from build123d import *

# Parameters (mm, degrees)
SKETCH1_W           = 92.252714028
SKETCH1_H           = 52.835645306
SKETCH1_R           = 8.1
BOSS_EXTRUDE1_DEPTH = 3
SKETCH2_R           = 11.1
SKETCH2_R_2         = 8.1
BOSS_EXTRUDE2_DEPTH = 2


with BuildPart() as part:
    # Sketch1 → Boss-Extrude1 (new body)
    with BuildSketch(Plane(origin=(0, 0, 0), x_dir=(1, 0, 0), z_dir=(0, 1, 0))):
        Rectangle(SKETCH1_W, SKETCH1_H)
        with Locations(Location((-25.470998192, 0, 0), (0, 0, 270))):
            Circle(SKETCH1_R, mode=Mode.SUBTRACT)
    extrude(amount=BOSS_EXTRUDE1_DEPTH)

    # Sketch2 → Boss-Extrude2 (add)
    with BuildSketch(Plane(origin=(0, 3, 0), x_dir=(1, 0, 0), z_dir=(0, 1, 0))):
        with Locations(Location((-25.470998192, 0, 0), (0, 0, 90))):
            Circle(SKETCH2_R)
        with Locations(Location((-25.470998192, 0, 0), (0, 0, 270))):
            Circle(SKETCH2_R_2, mode=Mode.SUBTRACT)
    extrude(amount=BOSS_EXTRUDE2_DEPTH)


solid = part.part
Work out the finished part from the listing and answer in its coordinate system (mm). Round coordinates to 2 decimals unless told otherwise and drop trailing zeros. Write each loop counter-clockwise with the first axis right and the second up, starting at its lowest first coordinate (ties: lowest second). Pieces come first, ordered by that corner, then holes.
1) The mould has two halves that part along Z. Classify faces 1 (the flat face through (-1, 1, -26.418)), 2 (the cylindrical face through (-14.635, 3.986, 2.406)), 3 (the cylindrical face through (-32.657, 2.465, 3.738)), 4 (the flat face through (-46.126, 1, 0)): pulls with the +Z half, pulls with the -Z half, needs draft (parallel to the pull), parting line crosses it, or undercut.
2) A cutting plane is placed at C-C (y = 2). Give the vertices of the cut face in (x, z), plus the area to 3 significant figures.
3) Given pin 1 Ø1.5 at (x, z) = (4.5, -9.5) entering from +Y; pin 2 Ø13 at (x, z) = (-25.47, 0) entering from -Y, each flat-ended and moving along its own axis, determine where each tip first touches the part or whether it passes through.
4) A cutting plane is placed at A-A (z = 0). Give the vertices of the cut face in (x, y), plus the area to 3 significant figures.
5) A cutting plane is placed at B-B (x = -32). Give the vertices of the cut face in (y, z).
6) A cutting plane is placed at D-D (z = 22). Give the vertices of the cut face in (x, y), plus the area to 3 significant figures.
7) Straight lines are drawn through the part: line 1 (X direction, y = 2.2, z = 0); line 2 (X direction, y = 3.5, z = 0); line 3 (Y direction, x = -19, z = -24). For each, find the intervals that lie inside material, in ascending order.
Completed:
1. face 1: pulls with the -Z half
1. face 2: parting line crosses it
1. face 3: undercut
1. face 4: needs draft
2. outline: (-46.13, -26.42) - (46.13, -26.42) - (46.13, 26.42) - (-46.13, 26.42) - close; hole circle Ø16.2 at (-25.47, 0)
2. area: 4,670 mm2
3. pin 1: stops at y = 3
3. pin 2: passes through
4. outline: (-46.13, 0) - (-33.57, 0) - (-33.57, 5) - (-36.57, 5) - (-36.57, 3) - (-46.13, 3) - close; (-17.37, 0) - (46.13, 0) - (46.13, 3) - (-14.37, 3) - (-14.37, 5) - (-17.37, 5) - close
4. area: 240 mm2
5. outline: (0, -26.42) - (3, -26.42) - (3, -8.98) - (5, -8.98) - (5, -4.79) - (0, -4.79) - close; (0, 4.79) - (5, 4.79) - (5, 8.98) - (3, 8.98) - (3, 26.42) - (0, 26.42) - close
6. outline: (-46.13, 0) - (46.13, 0) - (46.13, 3) - (-46.13, 3) - close
6. area: 277 mm2
7. line 1: x = -46.13 to -33.57, -17.37 to 46.13
7. line 2: x = -36.57 to -33.57, -17.37 to -14.37
7. line 3: y = 0 to 3
